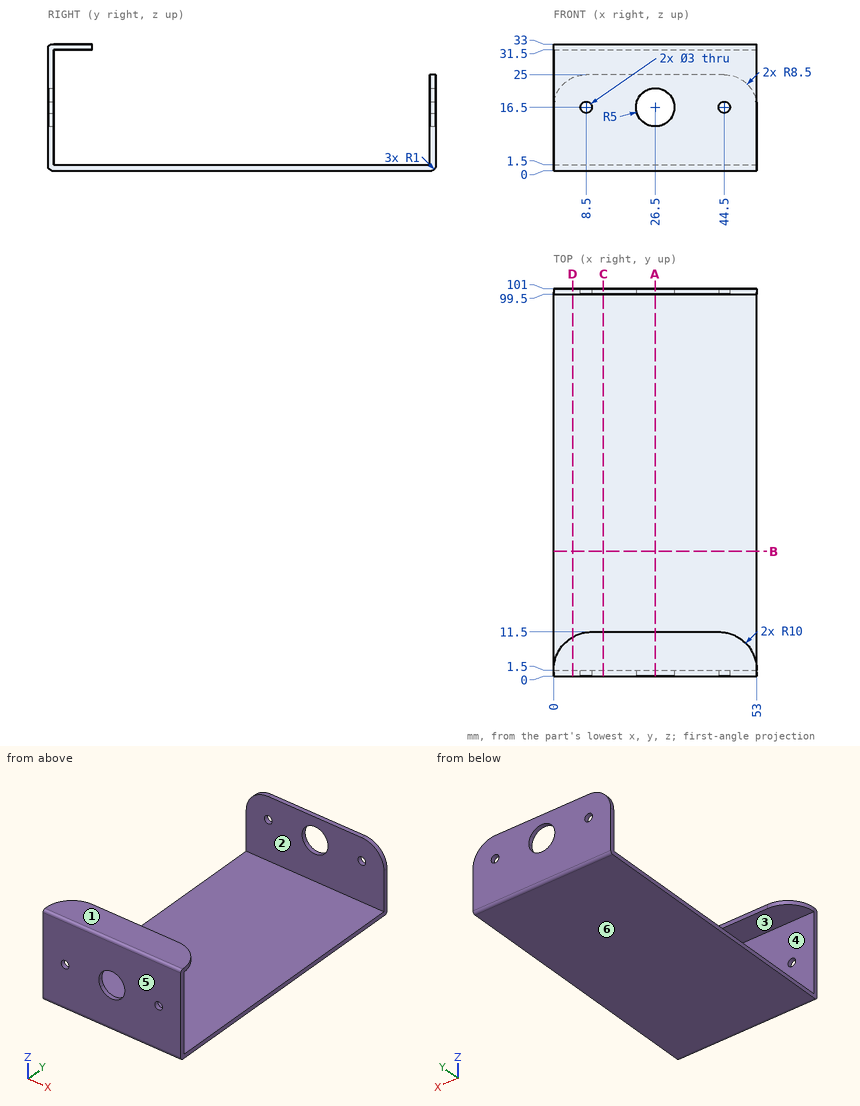
Design review of the part shown in the three views and the two pictorial views. Dimensions are in mm from the part's minimum x, y and z. A direction names the side the tool comes from. Give positions to 0.01 mm unless a question says otherwise; leave off trailing zeros. Loops run counter-clockwise (first coordinate to the right, second up) from the corner with the lowest first, then second, coordinate; pieces in that order, holes last. Notation, with made-up numbers: (75.25, 17) -> (114.25, 17) arc R22 ccw to (114.25, 38) -> close; hole circle Ø3 at (-27.75, 55.25). An arc over 180 degrees is marked (long way). One line per question, with ' | ' between items.
1) We need section D-D (x = 5). Write out the cut boundary in (y, z).
Resolved:
outline: (0, 1) arc R1 ccw to (1, 0) -> (100, 0) arc R1 ccw to (101, 1) -> (101, 24.25) -> (99.5, 24.25) -> (99.5, 1.5) -> (1.5, 1.5) -> (1.5, 31.5) -> (10.16, 31.5) -> (10.16, 33) -> (1, 33) arc R1 ccw to (0, 32) -> close
2) The part is to be moulded in two halves that separate along Z. For the marked faces 3, 4, 5 and 6, say which applies: +Z half, -Z half, draft (parallel to the pull), parting line (faces both ways), or undercut.
Resolved:
face 3: undercut | face 4: undercut | face 5: draft | face 6: -Z half
3) For the marked faces 1 and 2, list the 3-axis set-ups (+Z, -Z, +X, -X, +Y, -Y) from which the entire face can be reached by the end or side of a thin tool; tool diameter is ignored.
Resolved:
face 1: +Z, +X, -X, +Y, -Y | face 2: +Z, +X, -X
4) We need section B-B (y = 32.5). Write out the cut boundary in (x, z), plus the area to 3 significant figures.
Resolved:
outline: (0, 0) -> (53, 0) -> (53, 1.5) -> (0, 1.5) -> close | area: 79.5 mm2
5) Insertion check: pin 1 Ø0.8 at (x, z) = (33, 32.5) entering from +Y; pin 2 Ø1.6 at (x, y) = (22.5, 100.5) entering from +Z; pin 3 Ø16 at (x, y) = (22.5, 40) entering from +Z. Each pin has a flat end and moves straight along its axis. Give the tip position at first contact, or say it passes through.
Resolved:
pin 1: stops at y = 11.5 | pin 2: stops at z = 25 | pin 3: stops at z = 1.5
6) We need section C-C (x = 13). Write out the cut boundary in (y, z).
Resolved:
outline: (0, 1) arc R1 ccw to (1, 0) -> (100, 0) arc R1 ccw to (101, 1) -> (101, 25) -> (99.5, 25) -> (99.5, 1.5) -> (1.5, 1.5) -> (1.5, 31.5) -> (11.5, 31.5) -> (11.5, 33) -> (1, 33) arc R1 ccw to (0, 32) -> close
7) To check wall thickness, follow probe 1 along Y at (x, z) = (15, 10.5); probe 2 along Z at (x, y) = (18, 8.5); probe 3 along Z at (x, y) = (28, 64.5). State the ranges of each line that lie inside material, in increasing order.
Resolved:
probe 1: y = 0 to 1.5, 99.5 to 101 | probe 2: z = 0 to 1.5, 31.5 to 33 | probe 3: z = 0 to 1.5
8) We need section A-A (x = 26.5). Write out the cut boundary in (y, z).
Resolved:
outline: (0, 1) arc R1 ccw to (1, 0) -> (100, 0) arc R1 ccw to (101, 1) -> (101, 11.5) -> (99.5, 11.5) -> (99.5, 1.5) -> (1.5, 1.5) -> (1.5, 11.5) -> (0, 11.5) -> close; (0, 21.5) -> (1.5, 21.5) -> (1.5, 31.5) -> (11.5, 31.5) -> (11.5, 33) -> (1, 33) arc R1 ccw to (0, 32) -> close; (99.5, 21.5) -> (101, 21.5) -> (101, 25) -> (99.5, 25) -> close
